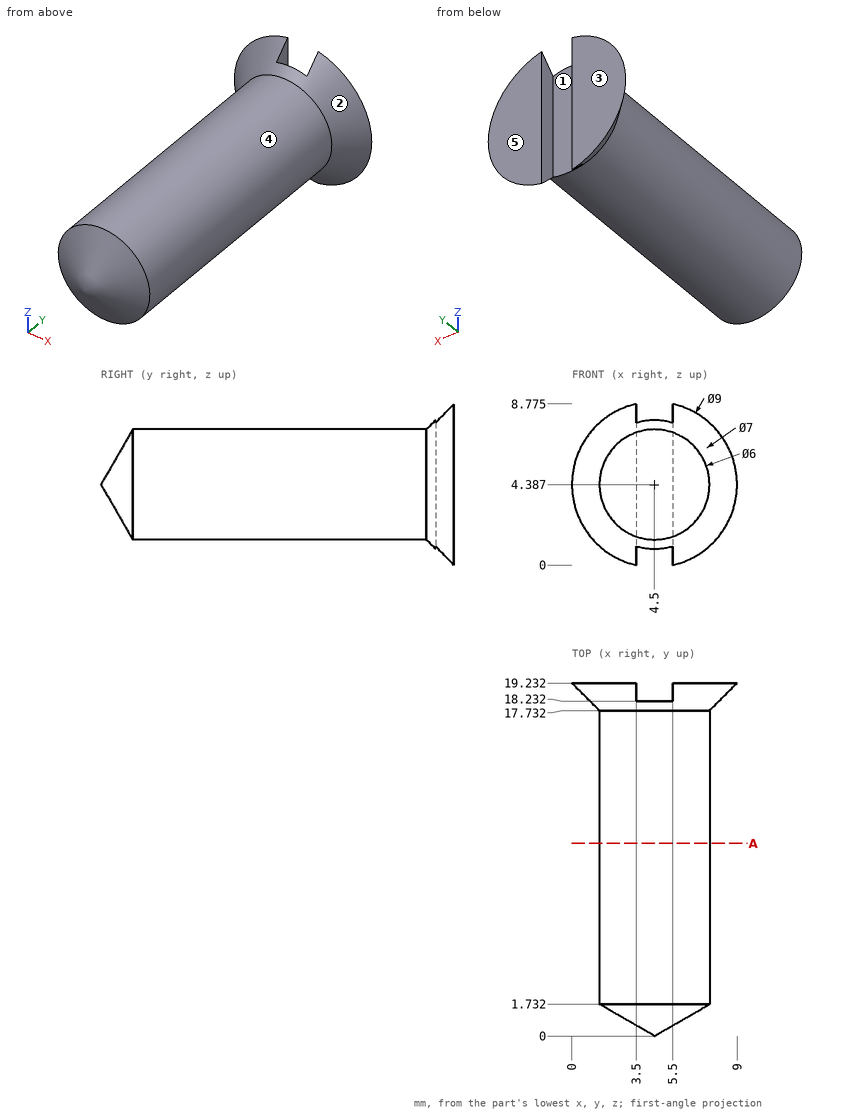
Geometry: see drawing. Coordinates: mm, zero at the bounding-box minimum. A direction names the side the tool comes from. Give positions to 0.01 mm unless a question says otherwise; leave off trailing zeros. Order: outer loops, then holes, each group sorted by start corner. A loop starts at its lowest first (then second) coordinate and runs counter-clockwise, first axis right, second up. Notation, with made-up numbers: (-17.5, 79) -> (35.5, 79) arc R25 ccw to (35.5, 117) -> close; hole circle Ø8 at (81.25, 22.25). An arc over 180 degrees is marked (long way). Write each question's results on one line, items separated by ' | '.
1) First-contact query: pin 1 Ø3 at (x, z) = (5, 6) entering from -Y; pin 2 Ø1 at (x, z) = (4.5, 3.5) entering from +Y; pin 3 Ø3 at (y, z) = (14.5, 8) entering from +X. Flat tips, straight axial feed; report the tip coordinate or a pass-through.
Geometry says:
pin 1: stops at y = 0.11 | pin 2: stops at y = 18.23 | pin 3: stops at x = 6.63
2) Cut plane A-A (y = 10.5). Output: boundary loops of the cut face in (x, z), and give its area (3 significant figures).
Geometry says:
outline: circle Ø6 at (4.5, 4.39) | area: 28.3 mm²
3) Set-up query: the marked faces 4 and 5. Return all of +Z, -Z, +X, -X, +Y, -Y with unobstructed straight access to the full face (end or side cutting, diameter ignored); none if empty.
Geometry says:
face 4: -Y | face 5: +Z, -Z, +X, -X, +Y
4) Draft query along X for the marked faces 1, 2 and 3. Return one class per face: released by +X, released by -X, zero draft, split by the parting line, or undercut.
Geometry says:
face 1: undercut | face 2: split by the parting line | face 3: zero draft
5) Line query: line 1 along X through (y, z) = (4.25, 4.5); line 2 along X through (y, z) = (16.75, 6); line 3 along Y through (x, z) = (6.25, 8.25) (1 decimal). Output: solid intervals per line, ascending.
Geometry says:
line 1: x = 1.5 to 7.5 | line 2: x = 1.97 to 7.03 | line 3: y = 19 to 19.2
